Check sheet for the modelled part. Datum: model origin and axes. Units: mm. Give positions to 0.01 mm unless a question says otherwise; leave off trailing zeros. Write each loop counter-clockwise with the first axis right and the second up, starting at its lowest first coordinate (ties: lowest second). Pieces come first, ordered by that corner, then holes. Notation, with made-up numbers: M 72,-16.5 L 89,-16.5 A25 ccw 89,1.5 Z; hole C -19.75,86 d4. An arc over 180 degrees is marked long. Use CSV: the item, a comma, the result in double quotes. Start each with the question number.
1. Cross-section at C-C, the plane z = 1.1. State how many separate pieces and enclosed holes the cut face has, and give its area (3 significant figures).
2. Scan lines: line 1 (Y direction, x = 35, z = 2.8) (3 decimals); line 2 (Y direction, x = 25.5, z = 0.75); line 3 (X direction, y = 7, z = 2.55). Record each from-to range of solid material in increasing order.
3. Cross-section at B-B, the plane x = 53. Enter the section's corners in (y, z), and give its area (3 significant figures).
4. Depth check by flat-ended pin: P1, Ø2, axis at x = 0.65, y = 0.53, coming from the -Z side; P2, Ø1, axis at x = 56, z = 0.5, coming from the +Y side; P3, Ø1.5, axis at y = 16, z = 2.5, coming from the +X side. Enter the tip coordinate at first touch or a pass-through.
5. Cross-section at A-A, the plane y = 9.5. Enter the section's corners in (x, z), and give its area (3 significant figures).
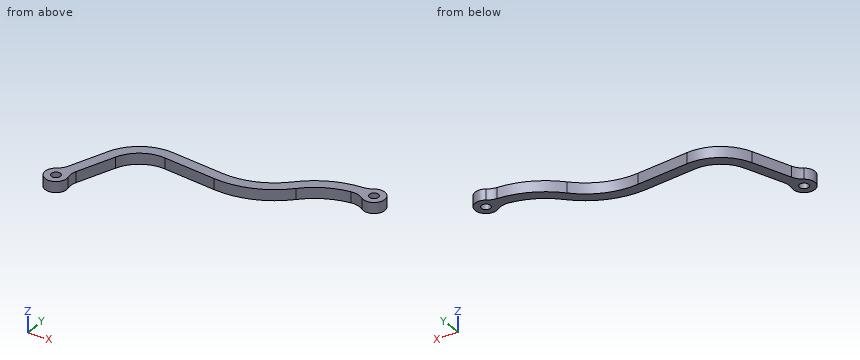
from build123d import *

# Parameters (mm, degrees)
EXTRUDE_THIN1_DEPTH   = 3
SKETCH1_3_R           = 3
BOSS_EXTRUDE1_DEPTH   = 3
FILLET1_R             = 5
F_2_5MM_DOWEL_HOLE1_D = 2.5


with BuildPart() as part:
    # Sketch1 → Extrude-Thin1 (new body)
    with BuildSketch(Plane.XY):
        with BuildLine():
            ThreePointArc((67.660273857, 34.169358704), (57.237958415, 33.249482811), (48.374242711, 27.690222541))
            ThreePointArc((48.374242711, 27.690222541), (41.120514889, 23.027861475), (32.560988498, 21.984460302))
            Line((32.560988498, 21.984460302), (18.0194176, 23.497567077))
            ThreePointArc((18.0194176, 23.497567077), (10.297542455, 21.776854665), (5.1667157, 15.754992513))
            Line((5.1667157, 15.754992513), (-0.737799909, 1.088733357))
            Line((-0.737799909, 1.088733357), (2.04513605, -0.031653828))
            Line((2.04513605, -0.031653828), (7.949651659, 14.634605328))
            ThreePointArc((7.949651659, 14.634605328), (11.845577871, 19.207110251), (17.7089323, 20.513677186))
            Line((17.7089323, 20.513677186), (32.250503198, 19.000570412))
            ThreePointArc((32.250503198, 19.000570412), (42.138725285, 20.205938799), (50.518449629, 25.592038399))
            ThreePointArc((50.518449629, 25.592038399), (58.193335463, 30.40567292), (67.217776658, 31.202172119))
            Line((67.217776658, 31.202172119), (67.660273857, 34.169358704))
        make_face()
    extrude(amount=EXTRUDE_THIN1_DEPTH)

    # Sketch1<3> → Boss-Extrude1 (add, through all)
    with BuildSketch(Plane.XY):
        with Locations((0.653668071, 0.528539764)):
            Circle(SKETCH1_3_R)
        with Locations((67.439025258, 32.685765412)):
            Circle(SKETCH1_3_R)
    extrude(amount=BOSS_EXTRUDE1_DEPTH)

    # Fillet1
    fillet1_edges = [part.edges().sort_by_distance(p)[0] for p in [
        (0.232483855, 3.498826595, 1.5),
        (3.015419815, 2.37843941, 1.5),
        (64.723514108, 31.410618677, 1.5),
        (64.980819062, 34.405423023, 1.5),
    ]]
    fillet(fillet1_edges, radius=FILLET1_R)

    # Ø2.5mm Dowel Hole1 (through all)
    with Locations(Plane.XY.offset(3)):
        with Locations((67.439025258, 32.685765412), (0.653668071, 0.528539764)):
            Hole(F_2_5MM_DOWEL_HOLE1_D / 2)


solid = part.part
Worked answers:
1,separate pieces,"1"
1,enclosed holes,"2"
1,area,"280 mm^2"
2,line 1,"y = 18.885 to 21.886"
2,line 2,"y = 19.7 to 22.72"
2,line 3,"x = 1.64 to 4.88"
3,outline,"M 27.73,0 L 31.31,0 L 31.31,3 L 27.73,3 Z"
3,area,"10.7 mm^2"
4,P1,"passes through"
4,P2,"stops at y = 32.99"
4,P3,"stops at x = 9.14"
5,outline,"M 2.65,0 L 5.88,0 L 5.88,3 L 2.65,3 Z"
5,area,"9.70 mm^2"
